For this review, use the dimensioned drawing (mm, ordinates from the lowest corner) and the shaded views. A direction names the side the tool comes from. Give positions to 0.01 mm unless a question says otherwise; leave off trailing zeros. Order: outer loops, then holes, each group sorted by start corner. A loop starts at its lowest first (then second) coordinate and runs counter-clockwise, first axis right, second up. Notation, with made-up numbers: M 9,54 L 37,54 A28 ccw 37,89 Z; hole C 31.25,-20 d7. An arc over 180 degrees is marked long. Answer as CSV lines item,"result". Start each with the question number.
1. We need section B-B, the plane x = 20. Give the boundary of the cut face in (y, z).
2. We need section A-A, the plane z = 5.25. Give the boundary of the cut face in (x, y).
3. For line 1 along X through (y, z) = (6.25, 5.25); line 2 along Y through (x, z) = (21.75, 4.75); line 3 along Z through (x, y) = (12, 5.5) (1 decimal), list the stretches that pass through material, from the lowest coordinate up.
4. We need section C-C, the plane y = 9.25. Give the boundary of the cut face in (x, z) (1 decimal).
5. Clearance check with flat-ended pins moving along their axes: P1, Ø6, axis at y = 5, z = 11.5, coming from the -X side; P2, Ø7.5, axis at x = 14.5, y = 12, coming from the +Z side (1 decimal); P3, Ø3.5, axis at y = 10.5, z = 5, coming from the +X side; P4, Ø8, axis at y = 10.5, z = 4.5, coming from the -X side. State where each tip first meets the part, or that it passes through.
6. Machinability: for the marked faces 1 and 2, which of the approach directions +Z, -Z, +X, -X, +Y, -Y give a long, thin tool a straight path to every point of the face, cutting with its end or side? Answer none if there is none.
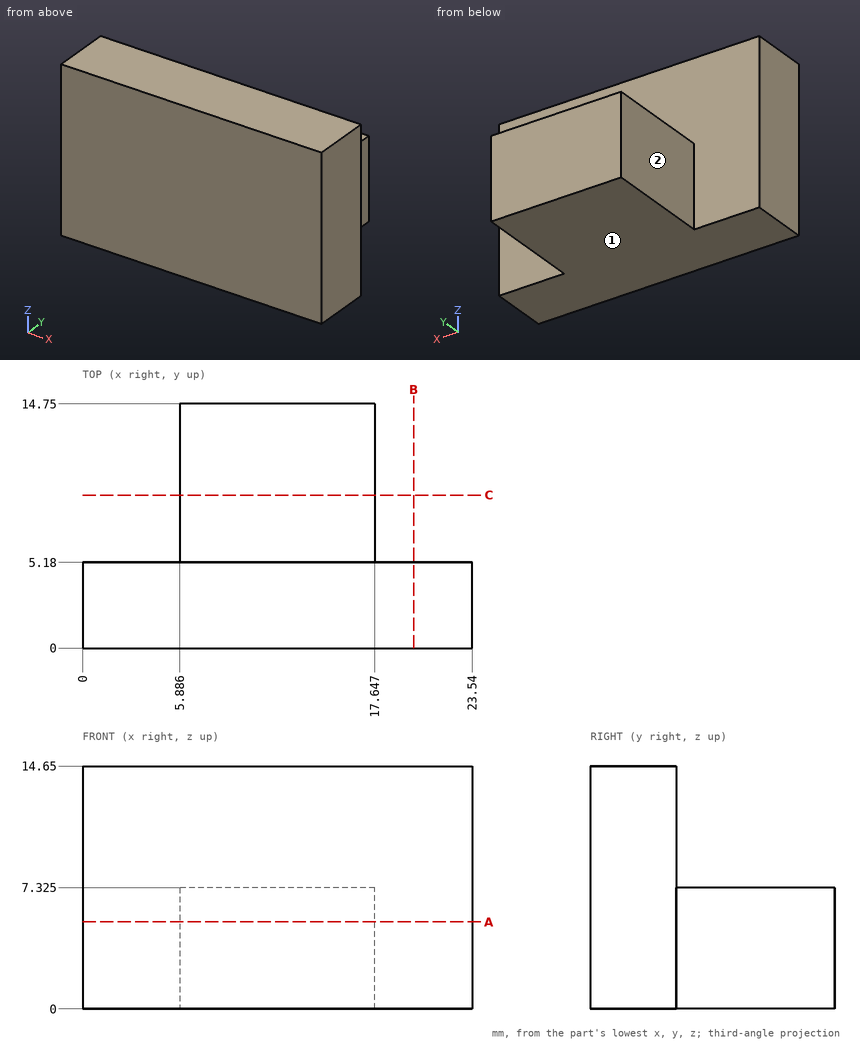
Result set:
1,outline,"M 0,0 L 5.18,0 L 5.18,14.65 L 0,14.65 Z"
2,outline,"M 0,0 L 23.54,0 L 23.54,5.18 L 17.65,5.18 L 17.65,14.75 L 5.89,14.75 L 5.89,5.18 L 0,5.18 Z"
3,line 1,"5.89 to 17.65"
3,line 2,"0 to 5.18"
3,line 3,"0 to 7.3"
4,outline,"M 5.9,0 L 17.6,0 L 17.6,7.3 L 5.9,7.3 Z"
5,P1,"x = 0"
5,P2,"z = 7.3"
5,P3,"x = 17.65"
5,P4,"x = 5.89"
6,face 1,"-Z, +X, -X, +Y, -Y"
6,face 2,"+Z, -Z, -X, +Y"
